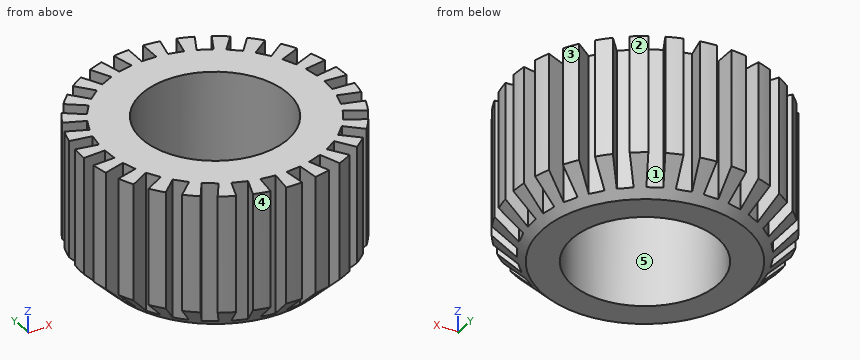
from build123d import *

# Parameters (mm, degrees)
SKETCH1_R           = 9
SKETCH1_R_2         = 5
BOSS_EXTRUDE1_DEPTH = 10
CHAMFER1_SIZE       = 2
CUT_EXTRUDE1_DEPTH  = 11
CIRPATTERN1_COUNT   = 27


with BuildPart() as part:
    # Sketch1 → Boss-Extrude1 (new body)
    with BuildSketch(Plane.XY):
        Circle(SKETCH1_R)
        Circle(SKETCH1_R_2, mode=Mode.SUBTRACT)
    extrude(amount=BOSS_EXTRUDE1_DEPTH)

    # Chamfer1
    chamfer1_edges = [part.edges().sort_by_distance(p)[0] for p in [
        (-9, 0, 0),
    ]]
    chamfer(chamfer1_edges, length=CHAMFER1_SIZE)

    # Sketch2 → Cut-Extrude1 (cut, through all)
    with BuildSketch(Plane(origin=(0, 0, 0), x_dir=(-1, 0, 0), z_dir=(0, 0, -1))):
        with BuildLine():
            Line((-0.5, 7.5), (0.5, 7.5))
            Line((0.5, 7.5), (0.5, 8.986100378))
            ThreePointArc((0.5, 8.986100378), (0, 9), (-0.5, 8.986100378))
            Line((-0.5, 8.986100378), (-0.5, 7.5))
        make_face()
    cut_extrude1 = extrude(amount=-CUT_EXTRUDE1_DEPTH, mode=Mode.SUBTRACT)

    # CirPattern1: Cut-Extrude1 ×27 about axis
    cirpattern1_axis = Axis((0, 0, 0), (0, 0, 1))
    for i in range(1, CIRPATTERN1_COUNT):
        add(cut_extrude1.rotate(cirpattern1_axis, i * 360 / CIRPATTERN1_COUNT), mode=Mode.SUBTRACT)


solid = part.part
Part model, mm, in its own coordinate system. Face numbers are marked on the shaded views. A direction names the side the tool comes from. Coordinates: 2 decimals unless noted, no trailing zeros. Loops run counter-clockwise (first coordinate to the right, second up) from the corner with the lowest first, then second, coordinate; pieces in that order, holes last. Notation, with made-up numbers: (-7.75, 73.5) - (4.25, 73.5) arc R23 ccw to (4.25, 106.5) - close; hole circle Ø10 at (-6, 24). An arc over 180 degrees is marked (long way). Write each question's results on one line, items separated by ' | '. Start each with the question number.
Q1. Probe line 1 along Y through (x, z) = (0, 4.25); line 2 along X through (y, z) = (-6.25, 9.25); line 3 along X through (y, z) = (3.25, 0.75). List the from-to ranges inside material, lowest first.
Q2. Drop flat-ended pins along their axis: pin 1 Ø0.5 at (x, z) = (0, 5) entering from +Y; pin 2 Ø2 at (x, z) = (-4, 8.5) entering from -Y; pin 3 Ø6 at (x, z) = (-5, 1) entering from -Y. Give the stop position or say it passes through.
Q3. Two-plate mould, pull along Y, no slides. Class the marked faces 3, 4 and 5: +Y half, -Y half, draft (parallel to the pull), parting line (faces both ways), or undercut.
Q4. Which spindle directions (+Z, -Z, +X, -X, +Y, -Y) get a long thin tool onto all of the face, cutting with end or side? Do the marked faces 1 and 2. Say none if no direction does.
Q5. Slice it at A-A on x = 0. Give the cut face in (y, z).
Answer:
1) line 1: y = -9 to -5, 5 to 7.5 | line 2: x = -5.9 to -4.71, -4.15 to 4.15, 4.71 to 5.9 | line 3: x = -6.77 to -3.8, 3.8 to 6.77
2) pin 1: stops at y = 7.5 | pin 2: stops at y = -8.27 | pin 3: stops at y = -8.73
3) face 3: +Y half | face 4: -Y half | face 5: undercut
4) face 1: +Z, -Z | face 2: +Z, -Z, +X, +Y
5) outline: (-9, 2) - (-7, 0) - (-5, 0) - (-5, 10) - (-9, 10) - close; (5, 0) - (7, 0) - (7.5, 0.5) - (7.5, 10) - (5, 10) - close
